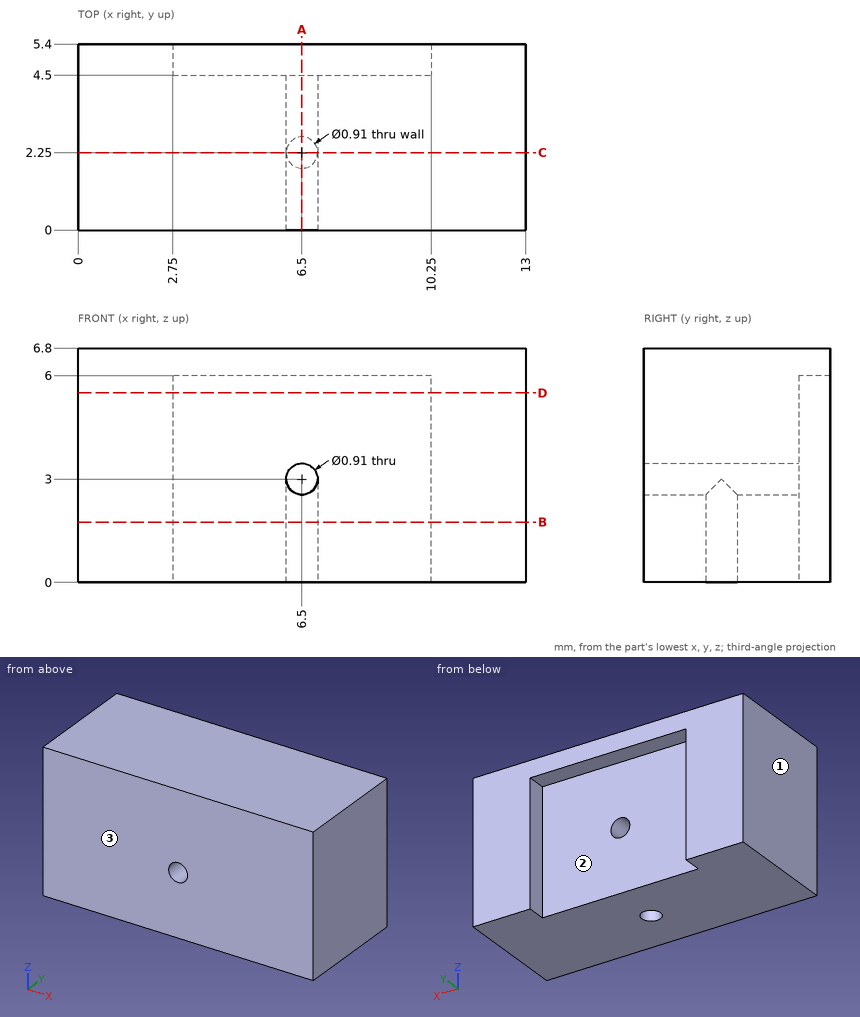
Geometry: see drawing. Coordinates: mm, zero at the bounding-box minimum. Give positions to 0.01 mm unless a question says otherwise; leave off trailing zeros. Order: outer loops, then holes, each group sorted by start corner. A loop starts at its lowest first (then second) coordinate and runs counter-clockwise, first axis right, second up.
Q1. Draft query along X for the marked faces 1, 2 and 3. Return one class per face: +X half, -X half, draft (parallel to the pull), parting line (faces both ways), or undercut.
Checked values:
face 1: -X half
face 2: undercut
face 3: draft
Q2. Ray query, probe 1 along Y at (x, z) = (5.25, 2); probe 2 along Z at (x, y) = (6, 4.7). Return the intervals inside material, ascending.
Checked values:
probe 1: y = 0 to 4.5
probe 2: z = 6 to 6.8
Q3. Section C-C on y = 2.25. Output: boundary loops of the cut face in (x, z) (3 decimals), and give its area (3 significant figures).
Checked values:
outline: (0, 0) - (6.045, 0) - (6.045, 3) arc R0.455 cw to (6.955, 3) - (6.955, 0) - (13, 0) - (13, 6.8) - (0, 6.8) - close
area: 85.3 mm2
Q4. Section D-D on z = 5.5. Output: boundary loops of the cut face in (x, y), and give its area (4 significant figures).
Checked values:
outline: (0, 0) - (13, 0) - (13, 5.4) - (10.25, 5.4) - (10.25, 4.5) - (2.75, 4.5) - (2.75, 5.4) - (0, 5.4) - close
area: 63.45 mm2
Q5. Contact query for flat-ended pins moving along their axis: pin 1 Ø1 at (x, z) = (4, 5) entering from +Y; pin 2 Ø0.5 at (x, y) = (6.5, 5) entering from -Z. Output: stop coordinate, or through.
Checked values:
pin 1: stops at y = 4.5
pin 2: stops at z = 6
Q6. Section A-A on x = 6.5. Output: boundary loops of the cut face in (y, z) (3 decimals), and give its area (3 significant figures).
Checked values:
outline: (0, 0) - (1.795, 0) - (1.795, 2.545) - (0, 2.545) - close; (0, 3.455) - (4.5, 3.455) - (4.5, 6) - (5.4, 6) - (5.4, 6.8) - (0, 6.8) - close; (2.705, 0) - (4.5, 0) - (4.5, 2.545) - (2.705, 2.545) - close
area: 24.9 mm2
Q7. Section B-B on z = 1.75. Output: boundary loops of the cut face in (x, y) (3 decimals).
Checked values:
outline: (0, 0) - (13, 0) - (13, 5.4) - (10.25, 5.4) - (10.25, 4.5) - (2.75, 4.5) - (2.75, 5.4) - (0, 5.4) - close; hole circle Ø0.91 at (6.5, 2.25)
